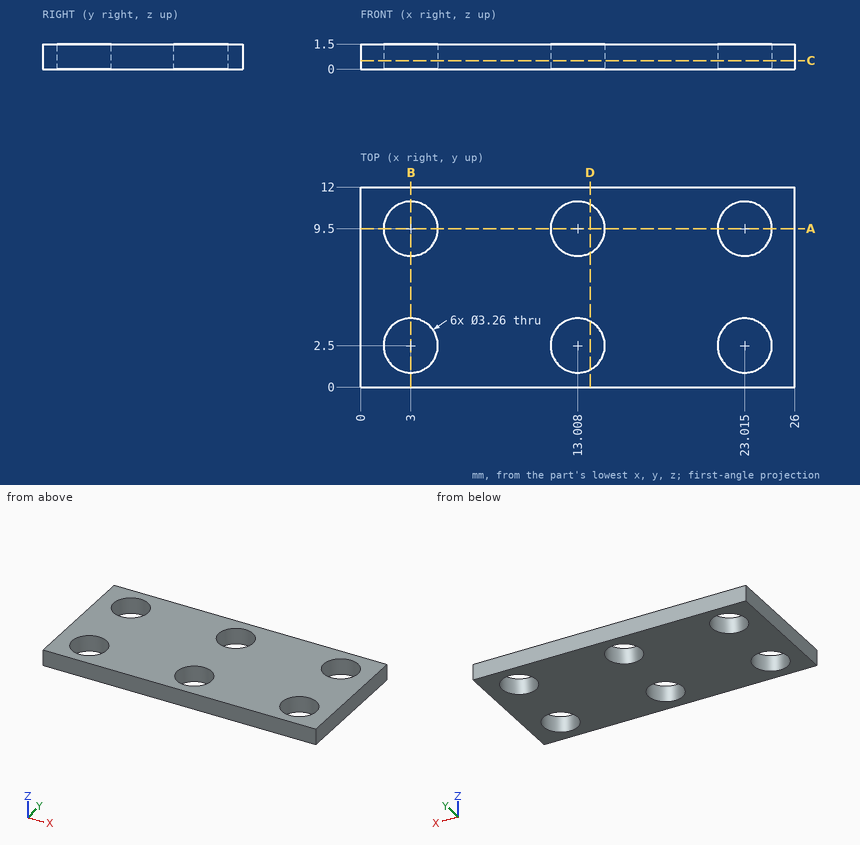
Geometry check sheet. Reference: drawing and pictorial views, mm from the part's lowest x, y, z. Give positions to 0.01 mm unless a question says otherwise; leave off trailing zeros. Loops run counter-clockwise (first coordinate to the right, second up) from the corner with the lowest first, then second, coordinate; pieces in that order, holes last. Notation, with made-up numbers: M 72.5,33.5 L 126.5,33.5 A14 cw 126.5,60.5 Z; hole C 0,35 d5. An arc over 180 degrees is marked long. Use a Markdown table: item, result. Add a question column.
Q1. Sectioned sample at C-C, the plane z = 0.5. Record the cut outline in (x, y) (1 decimal), then the cut area to 3 significant figures.
Q2. Sectioned sample at D-D, the plane x = 13.75. Record the cut outline in (y, z).
Q3. Sectioned sample at A-A, the plane y = 9.5. Record the cut outline in (x, z) (1 decimal).
Q4. Scan lines: line 1 along X through (y, z) = (9.5, 0.35) (1 decimal); line 2 along X through (y, z) = (9, 1.1) (1 decimal); line 3 along Y through (x, z) = (14.5, 1) (1 decimal). Record each from-to range of solid material in increasing order. Write a range as [from, to].
Q5. Sectioned sample at B-B, the plane x = 3. Record the cut outline in (y, z).
Verdict:
| question | item | result |
|---|---|---|
| 1 | outline | M 0,0 L 26,0 L 26,12 L 0,12 Z; hole C 3,2.5 d3.3; hole C 3,9.5 d3.3; hole C 13,2.5 d3.3; hole C 13,9.5 d3.3; hole C 23,2.5 d3.3; hole C 23,9.5 d3.3 |
| 1 | area | 262 mm^2 |
| 2 | outline | M 0,0 L 1.05,0 L 1.05,1.5 L 0,1.5 Z; M 3.95,0 L 8.05,0 L 8.05,1.5 L 3.95,1.5 Z; M 10.95,0 L 12,0 L 12,1.5 L 10.95,1.5 Z |
| 3 | outline | M 0,0 L 1.4,0 L 1.4,1.5 L 0,1.5 Z; M 4.6,0 L 11.4,0 L 11.4,1.5 L 4.6,1.5 Z; M 14.6,0 L 21.4,0 L 21.4,1.5 L 14.6,1.5 Z; M 24.6,0 L 26,0 L 26,1.5 L 24.6,1.5 Z |
| 4 | line 1 | [0, 1.4], [4.6, 11.4], [14.6, 21.4], [24.6, 26] |
| 4 | line 2 | [0, 1.4], [4.6, 11.5], [14.6, 21.5], [24.6, 26] |
| 4 | line 3 | [0, 1.8], [3.2, 8.8], [10.2, 12] |
| 5 | outline | M 0,0 L 0.87,0 L 0.87,1.5 L 0,1.5 Z; M 4.13,0 L 7.87,0 L 7.87,1.5 L 4.13,1.5 Z; M 11.13,0 L 12,0 L 12,1.5 L 11.13,1.5 Z |
